from build123d import *

# Parameters (mm, degrees)
SKETCH1_W           = 38.338603818
SKETCH1_H           = 9.300852407
BOSS_EXTRUDE1_DEPTH = 5


with BuildPart() as part:
    # Sketch1 → Boss-Extrude1 (new body)
    with BuildSketch(Plane.XY):
        with Locations((4.747182706, -0.026965663)):
            Rectangle(SKETCH1_W, SKETCH1_H)
        with BuildLine():
            Line((-8.377929756, 2.630922308), (-10.471711974, 1.422076581))
            ThreePointArc((-10.471711974, 1.422076581), (-11.077929756, 1.422076581), (-10.774820865, 0.897076581))
            Line((-10.774820865, 0.897076581), (-10.774820865, -1.520614872))
            ThreePointArc((-10.774820865, -1.520614872), (-11.077929756, -2.045614872), (-10.471711974, -2.045614872))
            Line((-10.471711974, -2.045614872), (-8.377929756, -3.254460599))
            ThreePointArc((-8.377929756, -3.254460599), (-8.074820865, -3.779460599), (-7.771711974, -3.254460599))
            Line((-7.771711974, -3.254460599), (-5.677929756, -2.045614872))
            ThreePointArc((-5.677929756, -2.045614872), (-5.071711974, -2.045614872), (-5.374820865, -1.520614872))
            Line((-5.374820865, -1.520614872), (-5.374820865, 0.897076581))
            ThreePointArc((-5.374820865, 0.897076581), (-5.071711974, 1.422076581), (-5.677929756, 1.422076581))
            Line((-5.677929756, 1.422076581), (-7.771711974, 2.630922308))
            ThreePointArc((-7.771711974, 2.630922308), (-8.074820865, 3.155922308), (-8.377929756, 2.630922308))
        make_face(mode=Mode.SUBTRACT)
        with BuildLine():
            Line((-0.303108891, 3.058161507), (-2.496891109, 1.791580754))
            ThreePointArc((-2.496891109, 1.791580754), (-3.103108891, 1.791580754), (-2.8, 1.266580754))
            Line((-2.8, 1.266580754), (-2.8, -1.266580754))
            ThreePointArc((-2.8, -1.266580754), (-3.103108891, -1.791580754), (-2.496891109, -1.791580754))
            Line((-2.496891109, -1.791580754), (-0.303108891, -3.058161507))
            ThreePointArc((-0.303108891, -3.058161507), (0, -3.583161507), (0.303108891, -3.058161507))
            Line((0.303108891, -3.058161507), (2.496891109, -1.791580754))
            ThreePointArc((2.496891109, -1.791580754), (3.103108891, -1.791580754), (2.8, -1.266580754))
            Line((2.8, -1.266580754), (2.8, 1.266580754))
            ThreePointArc((2.8, 1.266580754), (3.103108891, 1.791580754), (2.496891109, 1.791580754))
            Line((2.496891109, 1.791580754), (0.303108891, 3.058161507))
            ThreePointArc((0.303108891, 3.058161507), (0, 3.583161507), (-0.303108891, 3.058161507))
        make_face(mode=Mode.SUBTRACT)
        with BuildLine():
            Line((8.383417443, 3.171942265), (6.089635226, 1.847626484))
            ThreePointArc((6.089635226, 1.847626484), (5.483417443, 1.847626484), (5.786526334, 1.322626484))
            Line((5.786526334, 1.322626484), (5.786526334, -1.326005077))
            ThreePointArc((5.786526334, -1.326005077), (5.483417443, -1.851005077), (6.089635226, -1.851005077))
            Line((6.089635226, -1.851005077), (8.383417443, -3.175320858))
            ThreePointArc((8.383417443, -3.175320858), (8.686526334, -3.700320858), (8.989635226, -3.175320858))
            Line((8.989635226, -3.175320858), (11.283417443, -1.851005077))
            ThreePointArc((11.283417443, -1.851005077), (11.889635226, -1.851005077), (11.586526334, -1.326005077))
            Line((11.586526334, -1.326005077), (11.586526334, 1.322626484))
            ThreePointArc((11.586526334, 1.322626484), (11.889635226, 1.847626484), (11.283417443, 1.847626484))
            Line((11.283417443, 1.847626484), (8.989635226, 3.171942265))
            ThreePointArc((8.989635226, 3.171942265), (8.686526334, 3.696942265), (8.383417443, 3.171942265))
        make_face(mode=Mode.SUBTRACT)
        with BuildLine():
            Line((17.676043737, 3.17263624), (15.28226152, 1.790585433))
            ThreePointArc((15.28226152, 1.790585433), (14.676043737, 1.790585433), (14.979152629, 1.265585433))
            Line((14.979152629, 1.265585433), (14.979152629, -1.498516182))
            ThreePointArc((14.979152629, -1.498516182), (14.676043737, -2.023516182), (15.28226152, -2.023516182))
            Line((15.28226152, -2.023516182), (17.676043737, -3.40556699))
            ThreePointArc((17.676043737, -3.40556699), (17.979152629, -3.93056699), (18.28226152, -3.40556699))
            Line((18.28226152, -3.40556699), (20.676043737, -2.023516182))
            ThreePointArc((20.676043737, -2.023516182), (21.28226152, -2.023516182), (20.979152629, -1.498516182))
            Line((20.979152629, -1.498516182), (20.979152629, 1.265585433))
            ThreePointArc((20.979152629, 1.265585433), (21.28226152, 1.790585433), (20.676043737, 1.790585433))
            Line((20.676043737, 1.790585433), (18.28226152, 3.17263624))
            ThreePointArc((18.28226152, 3.17263624), (17.979152629, 3.69763624), (17.676043737, 3.17263624))
        make_face(mode=Mode.SUBTRACT)
    extrude(amount=BOSS_EXTRUDE1_DEPTH)


solid = part.part
Input: part model. Units: mm. Frame: model coordinates. A direction names the side the tool comes from. Round coordinates to 2 decimals unless told otherwise and drop trailing zeros. Order: outer loops, then holes, each group sorted by start corner. A loop starts at its lowest first (then second) coordinate and runs counter-clockwise, first axis right, second up. Notation, with made-up numbers: (66, 22) - (117, 22) arc R33 ccw to (117, 52) - close; hole circle Ø5 at (13.5, 84.5). An arc over 180 degrees is marked (long way). Answer as a JSON object with one key per item and string values. Group by question number.
(1) Material intervals for probe 1 along X at (y, z) = (0.5, 3); probe 2 along X at (y, z) = (3.5, 2.05); probe 3 along X at (y, z) = (3.25, 3.4), sorted ascending. Write a range as from..to.
(2) Cut plane B-B (z = 1.6). Count the separate pieces of the cut face and the enclosed holes in it, then the cut area to 3 significant figures.
(3) Cut plane A-A (y = 0). Return loops of the section in (x, z), then the cut area to 3 significant figures.
(4) Reachability of faces 5 (the face through (16.462, -2.705, 2.465)), 6 (the face through (4, 0, 5)) from +Z, -Z, +X, -X, +Y, -Y: full face, straight path, thin tool, end or side. Return the list, or none.
(5) Draft query along Y for faces 1 (the face through (20.979, 0, 2)), 2 (the face through (7.253, 2.519, 2.465)), 3 (the face through (4, 4.623, 2)), 4 (the face through (23.916, 0, 2)). Return one class per face: released by +Y, released by -Y, zero draft, split by the parting line, or undercut.
Here are the results:
{
 "1": {"probe 1": "x = -14.42..-10.77, -5.37..-2.8, 2.8..5.79, 11.59..14.98, 20.98..23.92", "probe 2": "x = -14.42..-0.23, 0.23..8.37, 9..17.66, 18.29..23.92", "probe 3": "x = -14.42..-0.35, 0.35..8.35, 9.02..17.64, 18.32..23.92"},
 "2": {"separate pieces": "1", "enclosed holes": "4", "area": "238 mm^2"},
 "3": {"outline": "(-14.42, 0) - (-10.77, 0) - (-10.77, 5) - (-14.42, 5) - close; (-5.37, 0) - (-2.8, 0) - (-2.8, 5) - (-5.37, 5) - close; (2.8, 0) - (5.79, 0) - (5.79, 5) - (2.8, 5) - close; (11.59, 0) - (14.98, 0) - (14.98, 5) - (11.59, 5) - close; (20.98, 0) - (23.92, 0) - (23.92, 5) - (20.98, 5) - close", "area": "77.7 mm^2"},
 "4": {"face 5": "+Z, -Z", "face 6": "+Z, +X, -X, +Y, -Y"},
 "5": {"face 1": "undercut", "face 2": "undercut", "face 3": "released by +Y", "face 4": "zero draft"}
}
